Autodesk Inventor part; units mm, degrees
ref_plane "YZ Plane" through (0, 0, 0) normal (1, 0, 0) x (0, 1, 0)
ref_plane "XZ Plane" through (0, 0, 0) normal (0, 1, 0) x (-1, 0, 0)
ref_plane "XY Plane" through (0, 0, 0) normal (0, 0, 1) x (1, 0, 0)
sketch "Sketch1" plane through (0, 0, 0) normal (0, 0, 1) x (1, 0, 0)
  line L0 (0, 0) -> (0, -40.9)
  line L1 (0, 0) -> (160, 0)
  line L2 (160, 0) -> (160, -40.9)
  line L3 (160, -40.9) -> (157.6, -40.9)
  line L4 (157.6, -40.9) -> (157.6, -2.4)
  line L5 (157.6, -2.4) -> (2.4, -2.4)
  line L6 (2.4, -2.4) -> (2.4, -40.9)
  line L7 (2.4, -40.9) -> (0, -40.9)
  line L8 (160, -21.65) -> (157.6, -21.65)
  line L9 (2.4, -21.65) -> (0, -21.65)
  dimension "d0" = 40.9
  dimension "d1" = 160
  dimension "d2" = 2.4
  dimension "d3" = 38.5
  dimension "d4" = 155.2
extrude "Extrusion5" add sketch "Sketch1" along normal blind 77.7 contours L9 L6 L7 L0 | L2 L3 L4 L8
extrude "Extrusion6" add sketch "Sketch1" along normal blind 10 contours L1 L2 L8 L4 L5 L6 L9 L0
sketch "Sketch6" plane through (160, -40.9, 77.7) normal (1, 0, 0) x (0, 0, -1)
  line L0 (0, 0) -> (0, 19.25)
  line L1 (0, 19.25) -> (0, 0)
  line L2 (77.7, 0) -> (0, 0)
  line L3 (0, 0) -> (-11.114, 19.25)
  line L4 (0, 0) -> (22.228, 0) construction
  line L5 (-11.114, 19.25) -> (0, 19.25)
  point P0 (77.7, 40.9)
  dimension "d21" = 120
extrude "Extrusion7" add sketch "Sketch6" against normal blind 2.4
sketch "Sketch7" plane through (0, -40.9, 77.7) normal (-1, 0, 0) x (0, 0, 1)
  line L0 (0, 0) -> (0, 19.25)
  line L1 (0, 19.25) -> (0, 0)
  line L2 (-67.7, 19.25) -> (11.114, 19.25)
  line L3 (0, 0) -> (11.114, 19.25)
  line L4 (11.114, 19.25) -> (0, 19.25)
  point P0 (-77.7, 40.9)
extrude "Extrusion8" add sketch "Sketch7" against normal blind 2.4
sketch "Sketch8" plane through (2.4, -40.9, 0) normal (1, 0, 0) x (0, 0, -1)
  line L0 (0, 0) -> (0, 2.4)
  line L1 (0, 0) -> (0, 38.5)
  line L2 (0, 2.4) -> (-79.0856, 2.4)
  line L3 (-88.814, 19.25) -> (-77.7, 0)
  line L4 (-77.7, 0) -> (0, 0)
  point P0 (0, 40.9)
  dimension "d26" = 2.4
extrude "Extrusion9" add sketch "Sketch8" along normal blind 157
sketch "Sketch9" plane through (2.4, -21.65, 10) normal (1, 0, 0) x (0, 0, -1)
  line L0 (10, -16.85) -> (10, 19.25)
  line L1 (10, -16.85) -> (10, -10.85)
  line L2 (10, -10.85) -> (7.6, -10.85)
  line L3 (7.6, -10.85) -> (7.6, -16.85)
  line L4 (-69.0856, -16.85) -> (10, -16.85)
  line L5 (7.6, -16.85) -> (10, -16.85)
  line L6 (-69.0856, -16.85) -> (-66.6856, -16.85)
  line L7 (-66.6856, -16.85) -> (-69.6856, -11.6538)
  line L8 (-69.6856, -11.6538) -> (-72.0856, -11.6538)
  line L9 (-67.7, -19.25) -> (-78.814, 0)
  line L10 (-72.0856, -11.6538) -> (-69.0856, -16.85)
  point P0 (10, 21.65)
  dimension "d29" = 6
  dimension "d30" = 2.4
  dimension "d31" = 6
  dimension "d32" = 90
  dimension "d33" = 2.4
  dimension "d34" = 6
  dimension "d35" = 60
  dimension "d36" = 120
extrude "Extrusion10" add sketch "Sketch9" along normal blind 157
sketch "Sketch10" plane through (0, -40.9, 0) normal (-1, 0, 0) x (0, 0, 1)
  line L0 (10, 40.9) -> (10, 19.25)
  line L1 (10, 19.25) -> (88.814, 19.25)
  line L2 (10, 19.25) -> (88.814, 19.25)
  line L3 (88.814, 19.25) -> (101.3136, 40.9)
  line L4 (88.814, 19.25) -> (113.8133, 19.25) construction
  line L5 (101.3136, 40.9) -> (10, 40.9)
  point P0 (0, 40.9)
  dimension "d39" = 60
extrude "Extrusion11" add sketch "Sketch10" against normal blind 2.4
sketch "Sketch11" plane through (160, -40.9, 0) normal (1, 0, 0) x (0, 0, -1)
  line L0 (-10, 40.9) -> (-10, 38.5)
  line L1 (-10, 40.9) -> (-10, 19.25)
  line L2 (-10, 19.25) -> (-88.814, 19.25)
  line L3 (-10, 19.25) -> (-88.814, 19.25)
  line L4 (-88.814, 19.25) -> (-101.3136, 40.9)
  line L5 (-101.3136, 40.9) -> (-10, 40.9)
  point P0 (0, 40.9)
extrude "Extrusion12" add sketch "Sketch11" against normal blind 2.4
properties part number "Chassi_Top_Rear"
Geometry: final body of the model. Coordinates: model frame, mm. A direction names the side the tool comes from. Coordinates: 2 decimals unless noted, no trailing zeros. Order: outer loops, then holes, each group sorted by start corner. A loop starts at its lowest first (then second) coordinate and runs counter-clockwise, first axis right, second up.
(1) Draft query along Y for faces 3 (the face through (0, -20, 50)), 4 (the face through (79, -35, 2.4)), 5 (the face through (81, -2.4, 5)), 6 (the face through (79, -40.9, 39)). Return one class per face: pulls with the +Y half, pulls with the -Y half, needs draft (parallel to the pull), parting line crosses it, or undercut.
(2) Access query for faces 1 (the face through (80, 0, 6)), 2 (the face through (78.914, -35.938, 78.165)). Directions: +Z, -Z, +X, -X, +Y, -Y. A direction counts if a zero-diameter tool reaches every point of the face in a straight line with its end or side. Return the directions, or none.
(3) Section query A-A (z = 37). Return the cut outline in (x, y).
(4) Section query D-D (z = 93). Return the cut outline in (x, y).
(5) Section query C-C (x = 28.5). Return the cut outline in (y, z).
(6) Material intervals for probe 1 along X at (y, z) = (-35.5, 12.5); probe 2 along Z at (x, y) = (10, -33.5); probe 3 along Y at (x, z) = (86, 21), sorted ascending.
(7) Section query B-B (y = -25). Return the cut outline in (x, z), plus the area to 3 significant figures.
(8) First-contact query: pin 1 (5 mm diameter, centred on x = 31.5, y = -30.5, fed in from +Z); pin 2 (1 mm diameter, centred on x = 96, y = -35, fed in from +Z); pin 3 (1.8 mm diameter, centred on x = 114, y = -35.5, fed in from +Z). Flat tips, straight axial feed; report the tip coordinate or a pass-through.
Solution:
1. face 3: needs draft
1. face 4: undercut
1. face 5: undercut
1. face 6: pulls with the -Y half
2. face 1: +Z, -Z, +X, -X, +Y
2. face 2: +Y
3. outline: (0, -40.9) - (160, -40.9) - (160, 0) - (157.6, 0) - (157.6, -38.5) - (2.4, -38.5) - (2.4, 0) - (0, 0) - close
4. outline: (0, -14.4) - (2.4, -14.4) - (2.4, 0) - (0, 0) - close; (157.6, -14.4) - (160, -14.4) - (160, 0) - (157.6, 0) - close
5. outline: (-40.9, 0) - (-32.5, 0) - (-32.5, 2.4) - (-38.5, 2.4) - (-38.5, 76.69) - (-33.3, 79.69) - (-33.3, 82.09) - (-40.9, 77.7) - close; (-2.4, 0) - (0, 0) - (0, 10) - (-2.4, 10) - close
6. probe 1: x = 0 to 2.4, 157.6 to 160
6. probe 2: z = 0 to 2.4, 79.57 to 81.97
6. probe 3: y = -40.9 to -38.5
7. outline: (0, 0) - (2.4, 0) - (2.4, 86.88) - (0, 86.88) - close; (157.6, 0) - (160, 0) - (160, 86.88) - (157.6, 86.88) - close
7. area: 417 mm2
8. pin 1: stops at z = 2.4
8. pin 2: stops at z = 81.4
8. pin 3: stops at z = 81.34
